Build history of the part. All positions in model axes, mm. A direction names the side the tool comes from. Round coordinates to 2 decimals unless told otherwise and drop trailing zeros. Loops run counter-clockwise (first coordinate to the right, second up) from the corner with the lowest first, then second, coordinate; pieces in that order, holes last. Notation, with made-up numbers: (43, 6.5) - (88, 6.5) arc R5 cw to (88, 11.5) - close; hole circle Ø7 at (-20.75, 62.25). An arc over 180 degrees is marked (long way). Put each result on its own line as item: value. Start each with the question number.
from build123d import *

# Parameters (mm, degrees)
SKETCH1_R                                        = 63.5
EXTRUDE1_DEPTH                                   = 32.7025
SKETCH2_R                                        = 38.1
CUT_EXTRUDE1_DEPTH                               = 33.7025
CUT_EXTRUDE2_DEPTH                               = 1.27
CUT_EXTRUDE3_DEPTH                               = 1.27
CBORE_FOR_1_2_SOCKET_HEAD_CAP_SCREW1_D           = 13.89126
CBORE_FOR_1_2_SOCKET_HEAD_CAP_SCREW1_CBORE_D     = 20.6375
CBORE_FOR_1_2_SOCKET_HEAD_CAP_SCREW1_CBORE_DEPTH = 13.97
F_1_2_20_TAPPED_HOLE1_AT_2_COUNT                 = 2
F_1_2_20_TAPPED_HOLE1_AT_2_PITCH                 = 87.988181024
F_1_2_20_TAPPED_HOLE1_AT_3_COUNT                 = 2
F_1_2_20_TAPPED_HOLE1_AT_3_PITCH                 = 87.988181024
CHAMFER1_SIZE                                    = 0.508


with BuildPart() as part:
    # Sketch1 → Extrude1 (new body)
    with BuildSketch(Plane.XY):
        with Locations(Location((0, 0, 0), (0, 0, 172.5))):  # turned: the seam where the file's is
            Circle(SKETCH1_R)
    extrude(amount=EXTRUDE1_DEPTH)

    # Sketch2 → Cut-Extrude1 (cut, through all)
    with BuildSketch(Plane.XY.offset(32.7025)):
        with Locations(Location((0, 0, 0), (0, 0, 7.5))):  # turned: the seam where the file's is
            Circle(SKETCH2_R)
    extrude(amount=-CUT_EXTRUDE1_DEPTH, mode=Mode.SUBTRACT)

    # Sketch3 → Cut-Extrude2 (cut)
    with BuildSketch(Plane.XY.offset(32.7025)):
        with BuildLine():
            Line((-38.656350742, 50.377937108), (-23.193810445, 30.226762265))
            ThreePointArc((-23.193810445, 30.226762265), (0, 38.1), (23.193810445, 30.226762265))
            Line((23.193810445, 30.226762265), (38.656350742, 50.377937108))
            ThreePointArc((38.656350742, 50.377937108), (0, 63.5), (-38.656350742, 50.377937108))
        make_face()
        with BuildLine():
            Line((-62.956748697, 8.288413206), (-37.774049218, 4.973047924))
            ThreePointArc((-37.774049218, 4.973047924), (-32.995567884, -19.05), (-14.580238773, -35.199810189))
            Line((-14.580238773, -35.199810189), (-24.300397955, -58.666350314))
            ThreePointArc((-24.300397955, -58.666350314), (-54.99261314, -31.75), (-62.956748697, 8.288413206))
        make_face()
        with BuildLine():
            Line((24.300397955, -58.666350314), (14.580238773, -35.199810189))
            ThreePointArc((14.580238773, -35.199810189), (32.995567884, -19.05), (37.774049218, 4.973047924))
            Line((37.774049218, 4.973047924), (62.956748697, 8.288413206))
            ThreePointArc((62.956748697, 8.288413206), (54.99261314, -31.75), (24.300397955, -58.666350314))
        make_face()
    extrude(amount=-CUT_EXTRUDE2_DEPTH, mode=Mode.SUBTRACT)

    # Sketch4 → Cut-Extrude3 (cut)
    with BuildSketch(Plane(origin=(0, 0, 0), x_dir=(-1, 0, 0), z_dir=(0, 0, -1))):
        with BuildLine():
            Line((24.300397955, -58.666350314), (14.580238773, -35.199810189))
            ThreePointArc((14.580238773, -35.199810189), (32.995567884, -19.05), (37.774049218, 4.973047924))
            Line((37.774049218, 4.973047924), (62.956748697, 8.288413206))
            ThreePointArc((62.956748697, 8.288413206), (54.99261314, -31.75), (24.300397955, -58.666350314))
        make_face()
        with BuildLine():
            Line((-24.300397955, -58.666350314), (-14.580238773, -35.199810189))
            ThreePointArc((-14.580238773, -35.199810189), (-32.995567884, -19.05), (-37.774049218, 4.973047924))
            Line((-37.774049218, 4.973047924), (-62.956748697, 8.288413206))
            ThreePointArc((-62.956748697, 8.288413206), (-54.99261314, -31.75), (-24.300397955, -58.666350314))
        make_face()
        with BuildLine():
            Line((-38.656350742, 50.377937108), (-23.193810445, 30.226762265))
            ThreePointArc((-23.193810445, 30.226762265), (0, 38.1), (23.193810445, 30.226762265))
            Line((23.193810445, 30.226762265), (38.656350742, 50.377937108))
            ThreePointArc((38.656350742, 50.377937108), (0, 63.5), (-38.656350742, 50.377937108))
        make_face()
    extrude(amount=-CUT_EXTRUDE3_DEPTH, mode=Mode.SUBTRACT)

    # CBORE for 1_2 Socket Head Cap Screw1 (through all)
    with Locations(Plane.XY.offset(31.4325)):
        with Locations((-43.994090512, -25.4), (0, 50.8), (43.994090512, -25.4)):
            CounterBoreHole(CBORE_FOR_1_2_SOCKET_HEAD_CAP_SCREW1_D / 2, CBORE_FOR_1_2_SOCKET_HEAD_CAP_SCREW1_CBORE_D / 2, CBORE_FOR_1_2_SOCKET_HEAD_CAP_SCREW1_CBORE_DEPTH)

    # Sketch9 → 1_2-20 Tapped Hole1 (revolve, cut)
    with BuildSketch(Plane(origin=(0, -50.8, 32.7025), x_dir=(0, -1, 0), z_dir=(1, 0, 0))):
        Polygon((0, 0), (0, 32.7025), (7.62, 32.7025), (6.35, 31.241532123), (6.35, 1.460967877), (7.62, 0), align=None)
    f_1_2_20_tapped_hole1 = revolve(axis=Axis((0, -50.8, 39.0525), (0, 0, -1)), mode=Mode.SUBTRACT)

    # 1_2-20 Tapped Hole1 at 2: 1_2-20 Tapped Hole1 ×2
    with Locations(*[Vector(-0.5, 0.866025404, 0) * (i * F_1_2_20_TAPPED_HOLE1_AT_2_PITCH) for i in range(1, F_1_2_20_TAPPED_HOLE1_AT_2_COUNT)]):
        add(f_1_2_20_tapped_hole1, mode=Mode.SUBTRACT)

    # 1_2-20 Tapped Hole1 at 3: 1_2-20 Tapped Hole1 ×2
    with Locations(*[Vector(0.5, 0.866025404, 0) * (i * F_1_2_20_TAPPED_HOLE1_AT_3_PITCH) for i in range(1, F_1_2_20_TAPPED_HOLE1_AT_3_COUNT)]):
        add(f_1_2_20_tapped_hole1, mode=Mode.SUBTRACT)

    # Chamfer1
    chamfer1_edges = [part.edges().sort_by_distance(p)[0] for p in [
        (-54.99261314, 31.75, 32.7025),
        (54.99261314, 31.75, 32.7025),
        (0, -63.5, 32.7025),
        (0, -63.5, 0),
        (54.99261314, 31.75, 0),
        (-54.99261314, 31.75, 0),
        (-50.365398958, 6.630730565, 0),
        (-50.365398958, 6.630730565, 32.7025),
        (-30.925080594, 40.302349687, 32.7025),
        (-32.995567884, 19.05, 32.7025),
        (30.925080594, 40.302349687, 32.7025),
        (50.365398958, 6.630730565, 32.7025),
        (32.995567884, 19.05, 32.7025),
        (19.440318364, -46.933080252, 32.7025),
        (-19.440318364, -46.933080252, 32.7025),
        (0, -38.1, 32.7025),
        (-19.440318364, -46.933080252, 0),
        (0, -38.1, 0),
        (19.440318364, -46.933080252, 0),
        (50.365398958, 6.630730565, 0),
        (30.925080594, 40.302349687, 0),
        (32.995567884, 19.05, 0),
        (-30.925080594, 40.302349687, 0),
        (-32.995567884, 19.05, 0),
    ]]
    chamfer(chamfer1_edges, length=CHAMFER1_SIZE)


solid = part.part
Item 1: Two-plate mould, pull along Y, no slides. Class faces 5 (the cylindrical face through (-37.055, -25.095, 9.253)), 6 (the flat face through (50.189, 6.608, 0.884)), 7 (the conical face through (-0.21, -38.24, 0.37)): pulls with the +Y half, pulls with the -Y half, needs draft (parallel to the pull), parting line crosses it, or undercut.
Item 2: Slice it at B-B (x = 0). Give the cut face in (y, z).
Item 3: Slice it at C-C (z = 29.5). Give the cut face in (x, y), plus the area to 3 significant figures.
Item 4: Which spindle directions (+Z, -Z, +X, -X, +Y, -Y) get a long thin tool onto all of the face, cutting with end or side? Do faces 1 (the flat face through (1, 43, 1.27)), 2 (the flat face through (-1, 40, 31.432)), 3 (the flat face through (-41, 33, 0)), 4 (the flat face through (39, -17, 1.27)). Say none if no direction does.
Item 5: Drop flat-ended pins along their axis: pin 1 Ø6 at (y, z) = (8.5, 16.5) entering from +X; pin 2 Ø2 at (y, z) = (42, 12) entering from +X; pin 3 Ø1.5 at (x, z) = (-31, 3.5) entering from +Y; pin 4 Ø20.5 at (x, y) = (0, -50.8) entering from +Z. Give the stop position or say it passes through.
Item 6: Slice it at D-D (y = -25.4). Give the cut face in (x, z).
Item 7: Drill centre lines: probe 1 along Y at (x, z) = (0, 26.5); probe 2 along Y at (x, z) = (0, 8.75); probe 3 along Y at (x, z) = (-42, 28). Where is each one in solid material? Low to high. Write a range as [from, to].
Item 8: Slice it at A-A (y = 0). Give the cut face in (x, z), plus the area to 3 significant figures.
Computed values:
1. face 5: undercut
1. face 6: pulls with the -Y half
1. face 7: pulls with the +Y half
2. outline: (-63.5, 0.51) - (-62.99, 0) - (-58.42, 0) - (-57.15, 1.46) - (-57.15, 31.24) - (-58.42, 32.7) - (-62.99, 32.7) - (-63.5, 32.19) - close; (-44.45, 1.46) - (-43.18, 0) - (-38.61, 0) - (-38.1, 0.51) - (-38.1, 32.19) - (-38.61, 32.7) - (-43.18, 32.7) - (-44.45, 31.24) - close; (38.1, 1.27) - (43.85, 1.27) - (43.85, 17.46) - (40.48, 17.46) - (40.48, 31.43) - (38.1, 31.43) - close; (57.75, 1.27) - (63.5, 1.27) - (63.5, 31.43) - (61.12, 31.43) - (61.12, 17.46) - (57.75, 17.46) - close
3. outline: circle Ø127 at (0, 0); hole circle Ø20.64 at (-43.99, -25.4); hole circle Ø12.7 at (-43.99, 25.4); hole circle Ø76.2 at (0, 0); hole circle Ø20.64 at (0, 50.8); hole circle Ø12.7 at (0, -50.8); hole circle Ø20.64 at (43.99, -25.4); hole circle Ø12.7 at (43.99, 25.4)
3. area: 6,720 mm^2
4. face 1: -Z, +Y
4. face 2: +Z, +Y
4. face 3: -Z, +X, -X, +Y, -Y
4. face 4: -Z, +X
5. pin 1: stops at x = 63.26
5. pin 2: stops at x = 48.49
5. pin 3: stops at y = 55.83
5. pin 4: stops at z = 32.7
6. outline: (-58.2, 1.27) - (-50.94, 1.27) - (-50.94, 17.46) - (-54.31, 17.46) - (-54.31, 31.43) - (-58.2, 31.43) - close; (-37.05, 1.27) - (-28.4, 1.27) - (-28.4, 31.43) - (-33.68, 31.43) - (-33.68, 17.46) - (-37.05, 17.46) - close; (28.4, 1.27) - (37.05, 1.27) - (37.05, 17.46) - (33.68, 17.46) - (33.68, 31.43) - (28.4, 31.43) - close; (50.94, 1.27) - (58.2, 1.27) - (58.2, 31.43) - (54.31, 31.43) - (54.31, 17.46) - (50.94, 17.46) - close
7. probe 1: y = [-63.5, -57.15], [-44.45, -38.1], [38.1, 40.48], [61.12, 63.5]
7. probe 2: y = [-63.5, -57.15], [-44.45, -38.1], [38.1, 43.85], [57.75, 63.5]
7. probe 3: y = [-47.63, -35.52], [-15.28, 19.37], [31.43, 47.63]
8. outline: (-63.5, 1.27) - (-38.1, 1.27) - (-38.1, 31.43) - (-63.5, 31.43) - close; (38.1, 1.27) - (63.5, 1.27) - (63.5, 31.43) - (38.1, 31.43) - close
8. area: 1,530 mm^2
